Verification items for the finished model (mm, model axes). A direction names the side the tool comes from. Coordinates: 2 decimals unless noted, no trailing zeros. Write each loop counter-clockwise with the first axis right and the second up, starting at its lowest first coordinate (ties: lowest second). Pieces come first, ordered by that corner, then holes. Notation, with made-up numbers: (-30, 23) - (21, 23) arc R25 ccw to (21, 55) - close; hole circle Ø10 at (-32.5, -35.5). An arc over 180 degrees is marked (long way). Answer as CSV lines item,"result". Start each with the question number.
```python
from build123d import *

# Parameters (mm, degrees)
ESQUISSE1_R             = 4
BOSS_EXTRU_1_DEPTH      = 6.35
ESQUISSE2_W             = 6.35
ESQUISSE2_H             = 15
ENL_V_MAT_EXTRU_1_DEPTH = 128.633547706
ESQUISSE3_R             = 12
ENL_V_MAT_EXTRU_2_DEPTH = 128.633547706


with BuildPart() as part:
    # Esquisse1 → Boss.-Extru.1 (new body)
    with BuildSketch(Plane(origin=(0, 0, 0), x_dir=(1, 0, 0), z_dir=(0, 1, 0))):
        with BuildLine():
            Line((-92.323711721, 55.00555093), (-17.323711721, -74.99444907))
            ThreePointArc((-17.323711721, -74.99444907), (0, -85), (17.323711721, -74.99444907))
            Line((17.323711721, -74.99444907), (92.323711721, 55.00555093))
            ThreePointArc((92.323711721, 55.00555093), (92.318905586, 75.00277508), (75, 85))
            Line((75, 85), (-75, 85))
            ThreePointArc((-75, 85), (-92.318905586, 75.00277508), (-92.323711721, 55.00555093))
        make_face()
        with Locations(Location((-75, 65, 0), (0, 0, 270))):
            Circle(ESQUISSE1_R, mode=Mode.SUBTRACT)
        with Locations(Location((75, 65, 0), (0, 0, 270))):
            Circle(ESQUISSE1_R, mode=Mode.SUBTRACT)
        with Locations(Location((0, -65, 0), (0, 0, 270))):
            Circle(ESQUISSE1_R, mode=Mode.SUBTRACT)
    extrude(amount=BOSS_EXTRU_1_DEPTH)

    # Esquisse2 → Enlèv. mat.-Extru.1 (cut, through all)
    with BuildSketch(Plane(origin=(0, 6.35, 0), x_dir=(1, 0, 0), z_dir=(0, 1, 0))):
        with Locations((0, -11.5)):
            Rectangle(ESQUISSE2_W, ESQUISSE2_H)
        with Locations((0, 13.5)):
            Rectangle(ESQUISSE2_W, ESQUISSE2_H)
        with Locations((0, -36.5)):
            Rectangle(ESQUISSE2_W, ESQUISSE2_H)
    extrude(amount=-ENL_V_MAT_EXTRU_1_DEPTH, mode=Mode.SUBTRACT)

    # Esquisse3 → Enlèv. mat.-Extru.2 (cut, through all)
    with BuildSketch(Plane(origin=(0, 6.35, 0), x_dir=(1, 0, 0), z_dir=(0, 1, 0))):
        with Locations(Location((0, 65, 0), (0, 0, 270))):
            Circle(ESQUISSE3_R)
    extrude(amount=-ENL_V_MAT_EXTRU_2_DEPTH, mode=Mode.SUBTRACT)


solid = part.part
```
1. Scan lines: line 1 along X through (y, z) = (2.25, -65); line 2 along X through (y, z) = (1.5, -62.5); line 3 along Z through (x, y) = (-3, 2.75). Record each from-to range of solid material in increasing order. Write a range as from..to.
2. Cross-section at A-A (y = 4). Record the cut outline in (x, z) (3 decimals), and give its area (3 significant figures).
3. Depth check by flat-ended pin: P1, Ø1.9, axis at y = 4.5, z = -11, coming from the -X side; P2, Ø3, axis at y = 1.5, z = -59, coming from the +X side; P3, Ø5, axis at x = 75, z = -65, coming from the -Y side; P4, Ø3, axis at x = 74.5, y = 3, coming from the +Z side. Enter the tip coordinate at first touch or a pass-through.
4. Cross-section at C-C (z = 35.5). Record the cut outline in (x, y) (3 decimals), and give its area (3 significant figures).
5. Cross-section at D-D (z = -65). Record the cut outline in (x, y).
6. Access from +Z, -Z, +X, -X, +Y, -Y to the whole of each face (thin tool, end or side, straight path). Record for faces 1 (the face through (-1, 0, -39)), 2 (the face through (0, 3, 19)).
7. Cross-section at B-B (x = 0). Record the cut outline in (y, z), and give its area (3 significant figures).
Completed:
1,line 1,"x = -95..-79, -71..-12, 12..71, 79..95"
1,line 2,"x = -94.84..-78.12, -71.88..-11.74, 11.74..71.88, 78.12..94.84"
1,line 3,"z = -85..-76.62, -53.38..-21, -6..4, 19..29, 44..62.35, 67.65..84.77"
2,outline,"(-92.324, -55.006) arc R20 ccw to (-75, -85) - (75, -85) arc R20 ccw to (92.324, -55.006) - (17.324, 74.994) arc R20 ccw to (-17.324, 74.994) - close; hole circle Ø8 at (-75, -65); hole circle Ø24 at (0, -65); hole circle Ø8 at (0, 65); hole (-3.175, -21) - (3.175, -21) - (3.175, -6) - (-3.175, -6) - close; hole (-3.175, 4) - (3.175, 4) - (3.175, 19) - (-3.175, 19) - close; hole (-3.175, 29) - (3.175, 29) - (3.175, 44) - (-3.175, 44) - close; hole circle Ø8 at (75, -65)"
2,area,"19,100 mm2"
3,P1,"stops at x = -67.48"
3,P2,"stops at x = 94.49"
3,P3,"passes through"
3,P4,"stops at z = -21.51"
4,outline,"(-40.109, 0) - (-3.175, 0) - (-3.175, 6.35) - (-40.109, 6.35) - close; (3.175, 0) - (40.109, 0) - (40.109, 6.35) - (3.175, 6.35) - close"
4,area,"469 mm2"
5,outline,"(-95, 0) - (-79, 0) - (-79, 6.35) - (-95, 6.35) - close; (-71, 0) - (-12, 0) - (-12, 6.35) - (-71, 6.35) - close; (12, 0) - (71, 0) - (71, 6.35) - (12, 6.35) - close; (79, 0) - (95, 0) - (95, 6.35) - (79, 6.35) - close"
6,face 1,"+Z, -Z, +X, -X, -Y"
6,face 2,"+Y, -Y"
7,outline,"(0, -85) - (6.35, -85) - (6.35, -77) - (0, -77) - close; (0, -53) - (6.35, -53) - (6.35, -21) - (0, -21) - close; (0, -6) - (6.35, -6) - (6.35, 4) - (0, 4) - close; (0, 19) - (6.35, 19) - (6.35, 29) - (0, 29) - close; (0, 44) - (6.35, 44) - (6.35, 61) - (0, 61) - close; (0, 69) - (6.35, 69) - (6.35, 85) - (0, 85) - close"
7,area,"591 mm2"
